```python
from build123d import *

# Parameters (mm, degrees)
F1_DEPTH = 10
F2_W     = 9
F2_H     = 2
F3_DEPTH = 8
F4_R     = 1.3
F5_DEPTH = 2


# Not quite as in the source:
# - a feature names something its author has since deleted; it is built from what else it names


with BuildPart() as f1:
    # F0 (on Top) → F1 (new body)
    with BuildSketch(Plane.XY):
        Polygon((-5, -6.5), (5, -6.5), (5, 6.5), (-5, 6.5), (-5, 4.5), (-3, 4.5), (3, 4.5), (3, -4.5), (-3, -4.5), (-5, -4.5), align=None)
    extrude(amount=F1_DEPTH)

    # F2 (on face) → F3 (join)
    with BuildSketch(Plane(origin=(3, 0, 0), x_dir=(0, -1, 0), z_dir=(-1, 0, 0))):
        with Locations((0, 1)):
            Rectangle(F2_W, F2_H)
    extrude(amount=F3_DEPTH)

    # F4 (on face) → F5 (cut, through all)
    with BuildSketch(Plane.XZ.offset(6.5)):
        with Locations((-1, 6)):
            Circle(F4_R)
    extrude(amount=-F5_DEPTH, mode=Mode.SUBTRACT)


solid = f1.part
```
Build history of the part. All positions in model axes, mm. A direction names the side the tool comes from. Round coordinates to 2 decimals unless told otherwise and drop trailing zeros. Loops run counter-clockwise (first coordinate to the right, second up) from the corner with the lowest first, then second, coordinate; pieces in that order, holes last.
Item 1: Saw through at D-D (x = 1). List the corners of the cut face in (y, z), then the cut area to 3 significant figures.
Item 2: Two-plate mould, pull along X, no slides. Class faces 1 (the face through (5, 0, 5)), 2 (the face through (-1.28, -5.51, 4.73)), 3 (the face through (0, -6.5, 4)): released by +X, released by -X, zero draft, split by the parting line, or undercut.
Item 3: Saw through at C-C (y = -5.5). List the corners of the cut face in (x, z).
Item 4: Drill centre lines: line 1 along Y through (x, z) = (1.75, 9); line 2 along Z through (x, y) = (-1, -6); line 3 along X through (y, z) = (-1.25, 6.5). Where is each one in solid material? Low to high.
Item 5: Which spindle directions (+Z, -Z, +X, -X, +Y, -Y) get a long thin tool onto all of the face, cutting with end or side? Do faces 4 (the face through (-1, 4.5, 6)), 5 (the face through (-5, 0.1, 1.7)). Say none if no direction does.
Item 6: Saw through at A-A (z = 6). List the corners of the cut face in (x, y), then the cut area to 3 significant figures.
Item 7: Saw through at B-B (x = -1). List the corners of the cut face in (y, z).
Item 8: Pin check, flat tips, straight feed: P1, Ø3, axis at y = 2.5, z = 5.5, coming from the -X side; P2, Ø4, axis at x = -0.5, y = -1, coming from the +Z side. Stop position of each tip, or through.
Worked answers:
1. outline: (-6.5, 0) - (6.5, 0) - (6.5, 10) - (4.5, 10) - (4.5, 2) - (-4.5, 2) - (-4.5, 10) - (-6.5, 10) - close
1. area: 58.0 mm2
2. face 1: released by +X
2. face 2: undercut
2. face 3: zero draft
3. outline: (-5, 0) - (5, 0) - (5, 10) - (-5, 10) - close; hole circle Ø2.6 at (-1, 6)
4. line 1: y = -6.5 to -4.5, 4.5 to 6.5
4. line 2: z = 0 to 4.7, 7.3 to 10
4. line 3: x = 3 to 5
5. face 4: +Z, -X
5. face 5: +Z, -Z, -X, +Y, -Y
6. outline: (-5, -6.5) - (-2.3, -6.5) - (-2.3, -4.5) - (-5, -4.5) - close; (-5, 4.5) - (3, 4.5) - (3, -4.5) - (0.3, -4.5) - (0.3, -6.5) - (5, -6.5) - (5, 6.5) - (-5, 6.5) - close
6. area: 52.8 mm2
7. outline: (-6.5, 0) - (6.5, 0) - (6.5, 10) - (4.5, 10) - (4.5, 2) - (-4.5, 2) - (-4.5, 4.7) - (-6.5, 4.7) - close; (-6.5, 7.3) - (-4.5, 7.3) - (-4.5, 10) - (-6.5, 10) - close
8. P1: stops at x = 3
8. P2: stops at z = 2
